Model file for the job. Use its own axes, mm. A direction names the side the tool comes from. Give positions to 0.01 mm unless a question says otherwise; leave off trailing zeros. Loops run counter-clockwise (first coordinate to the right, second up) from the corner with the lowest first, then second, coordinate; pieces in that order, holes last. Notation, with made-up numbers: M 74,37 L 86,37 A26 cw 86,59 Z; hole C 31,-21 d6. An arc over 180 degrees is marked long. Answer in a Markdown table with one row per item.
```python
from build123d import *

# Parameters (mm, degrees)
F0_W      = 68.1
F0_H      = 138.3
F1_DEPTH  = 5.08
F2_R      = 8.93259
F3_T      = -1.15
F4_W      = 24.09836
F4_H      = 13.196725
F5_DEPTH  = 12.5
F6_W      = 48.097777
F6_H      = 7.753484
F7_DEPTH  = 12.5
F8_W      = 10.118616
F8_H      = 41.666549
F9_DEPTH  = 12.5
F10_W     = 6.856616
F10_H     = 19.977162
F11_DEPTH = 12.5
F12_SIZE  = 5
F14_DEPTH = 25
F16_DEPTH = 25


with BuildPart() as f1:
    # F0 (on Front) → F1 (new body, symmetric)
    with BuildSketch(Plane.XZ):
        Rectangle(F0_W, F0_H)
    extrude(amount=F1_DEPTH, both=True)

    # F2
    f2_edges = [f1.edges().sort_by_distance(p)[0] for p in [
        (-34.05, 0, 69.15),
        (34.05, 0, 69.15),
        (34.05, 0, -69.15),
        (-34.05, 0, -69.15),
    ]]
    fillet(f2_edges, radius=F2_R)

    # F3
    f3_openings = [f1.faces().sort_by_distance(p)[0] for p in [
        (0, -5.08, 0),
    ]]
    offset(amount=F3_T, openings=f3_openings)

    # F4 (on face) → F5 (cut, symmetric)
    with BuildSketch(Plane.XZ):
        with Locations((15.348363, 59.815576)):
            Rectangle(F4_W, F4_H)
    extrude(amount=F5_DEPTH, both=True, mode=Mode.SUBTRACT)

    # F6 (on face) → F7 (cut, symmetric)
    with BuildSketch(Plane(origin=(0, 0, -69.15), x_dir=(1, 0, 0), z_dir=(0, 0, -1))):
        with Locations((0.003194, 0.064824)):
            Rectangle(F6_W, F6_H)
    extrude(amount=F7_DEPTH, both=True, mode=Mode.SUBTRACT)

    # F8 (on face) → F9 (cut, symmetric)
    with BuildSketch(Plane(origin=(-34.05, 0, 0), x_dir=(0, -1, 0), z_dir=(-1, 0, 0))):
        with Locations((3.675346, 37.227889)):
            Rectangle(F8_W, F8_H)
    extrude(amount=F9_DEPTH, both=True, mode=Mode.SUBTRACT)

    # F10 (on face) → F11 (cut, symmetric)
    with BuildSketch(Plane.YZ.offset(34.05)):
        with Locations((-1.651692, 39.359077)):
            Rectangle(F10_W, F10_H)
    extrude(amount=F11_DEPTH, both=True, mode=Mode.SUBTRACT)

    # F12
    f12_edges = [f1.edges().sort_by_distance(p)[0] for p in [
        (3.299183, 4.505, 66.413939),
        (27.397543, 4.505, 66.413939),
        (27.397543, 4.505, 53.217214),
        (3.299183, 4.505, 53.217214),
    ]]
    chamfer(f12_edges, length=F12_SIZE)

    # F13 (on face) → F14 (cut)
    with BuildSketch(Plane(origin=(0, 5.08, 0), x_dir=(-1, 0, 0), z_dir=(0, 1, 0))):
        with BuildLine():
            Line((-27.397543, 61.413939), (-22.397543, 66.413939))
            ThreePointArc((-22.397543, 66.413939), (-27.728042, 59.815576), (-22.397543, 53.217214))
            Line((-22.397543, 53.217214), (-27.397543, 58.217214))
            Line((-27.397543, 58.217214), (-27.397543, 61.413939))
        make_face()
    extrude(amount=-F14_DEPTH, mode=Mode.SUBTRACT)

    # F15 (on face) → F16 (cut)
    with BuildSketch(Plane(origin=(0, 5.08, 0), x_dir=(-1, 0, 0), z_dir=(0, 1, 0))):
        with BuildLine():
            Line((-3.299183, 58.217214), (-8.299183, 53.217214))
            ThreePointArc((-8.299183, 53.217214), (-1.70082, 59.815576), (-8.299183, 66.413939))
            Line((-8.299183, 66.413939), (-3.299183, 61.413939))
            Line((-3.299183, 61.413939), (-3.299183, 58.217214))
        make_face()
    extrude(amount=-F16_DEPTH, mode=Mode.SUBTRACT)


solid = f1.part
```
(1) Saw through at A-A, the plane x = -13. Give the cut face in (y, z), and give its area (3 significant figures).
Established:
| item | result |
|---|---|
| outline | M -5.08,-69.15 L -3.94,-69.15 L -3.94,-68 L -5.08,-68 Z; M -5.08,68 L 3.93,68 L 3.93,-68 L 3.81,-68 L 3.81,-69.15 L 5.08,-69.15 L 5.08,69.15 L -5.08,69.15 Z |
| area | 171 mm2 |
(2) Which spindle directions (+Z, -Z, +X, -X, +Y, -Y) get a long thin tool onto all of the face, cutting with end or side? Do faces 5 (the cylindrical face through (27.727, 4.513, 59.944)), 6 (the cylindrical face through (30.68, -0.51, 65.66)), 7 (the flat face through (0, 5.08, 1)). Say none if no direction does.
Established:
| item | result |
|---|---|
| face 5 | +Y, -Y |
| face 6 | -Y |
| face 7 | +Z, -Z, +X, -X, +Y |
(3) Saw through at D-D, the plane z = 3. Give the cut face in (x, y).
Established:
| item | result |
|---|---|
| outline | M -34.05,-5.08 L -32.9,-5.08 L -32.9,3.93 L 32.9,3.93 L 32.9,-5.08 L 34.05,-5.08 L 34.05,5.08 L -34.05,5.08 Z |
(4) Saw through at B-B, the plane y = -1.25. Give the cut face in (x, z), and give its area (3 significant figures).
Established:
| item | result |
|---|---|
| outline | M -34.05,-60.22 A8.93 ccw -25.12,-69.15 L -24.05,-69.15 L -24.05,-68 L -25.12,-68 A7.78 cw -32.9,-60.22 L -32.9,16.39 L -34.05,16.39 Z; M -34.05,58.06 L -32.9,58.06 L -32.9,60.22 A7.78 cw -25.12,68 L 25.12,68 A7.78 cw 32.9,60.22 L 32.9,49.35 L 34.05,49.35 L 34.05,60.22 A8.93 ccw 25.12,69.15 L -25.12,69.15 A8.93 ccw -34.05,60.22 Z; M 24.05,-69.15 L 25.12,-69.15 A8.93 ccw 34.05,-60.22 L 34.05,29.37 L 32.9,29.37 L 32.9,-60.22 A7.78 cw 25.12,-68 L 24.05,-68 Z |
| area | 327 mm2 |
(5) Wall check: L1, parallel to X at y = -0.75, z = 8.5; L2, parallel to Z at x = 25, y = -0.25; L3, parallel to Z at x = 25.5, y = 3.25. Give the ranges that are in metal, low to high.
Established:
| item | result |
|---|---|
| L1 | x = -34.05 to -32.9, 32.9 to 34.05 |
| L2 | z = -69.15 to -68, 68 to 69.15 |
| L3 | z = -69.14 to -67.99, 67.99 to 69.14 |
(6) Saw through at C-C, the plane x = 5. Give the cut face in (y, z).
Established:
| item | result |
|---|---|
| outline | M -5.08,-69.15 L -3.94,-69.15 L -3.94,-68 L -5.08,-68 Z; M -5.08,68 L 3.93,68 L 3.93,65.53 L 5.08,65.53 L 5.08,69.15 L -5.08,69.15 Z; M 3.81,-69.15 L 5.08,-69.15 L 5.08,54.1 L 3.93,54.1 L 3.93,-68 L 3.81,-68 Z |
(7) Flat gauge pins, fed straight in: P1, Ø3, axis at x = -8.5, z = -32, coming from the -Y side; P2, Ø0.6, axis at x = -33.5, z = 47, coming from the -Y side; P3, Ø1, axis at x = 26, y = -4, coming from the -Z side. Where does each tip first touch, or does it go through?
Established:
| item | result |
|---|---|
| P1 | stops at y = 3.93 |
| P2 | stops at y = 1.38 |
| P3 | stops at z = -69.14 |
(8) Mould opens along Z. For faces 1 (the flat face through (-0.1, -4.3, -68)), 2 (the flat face through (32.9, -1, -1)), 3 (the flat face through (0, 0, 69.15)), 4 (the flat face through (34.05, 0, -1)) say: pulls with the +Z half, pulls with the -Z half, needs draft (parallel to the pull), parting line crosses it, or undercut.
Established:
| item | result |
|---|---|
| face 1 | undercut |
| face 2 | undercut |
| face 3 | pulls with the +Z half |
| face 4 | needs draft |
